The drawing under review shows one solid part. Ordinate dimensions are in mm from its lowest x, y, z. Round coordinates to 2 decimals unless told otherwise and drop trailing zeros. Write each loop counter-clockwise with the first axis right and the second up, starting at its lowest first coordinate (ties: lowest second). Pieces come first, ordered by that corner, then holes. Notation, with made-up numbers: (86.5, 61.5) -> (138.5, 61.5) arc R20 cw to (138.5, 86.5) -> close; hole circle Ø8 at (45.25, 70.5). An arc over 180 degrees is marked (long way). Write item = value, one per line. Start each with the question number.
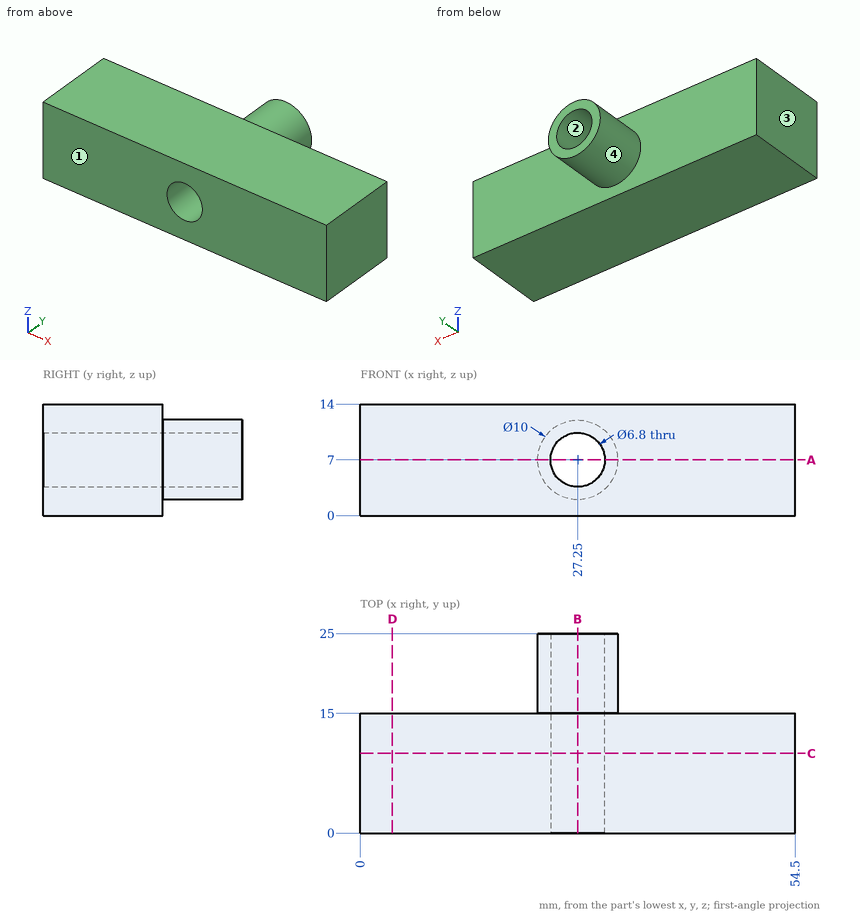
1. Draft analysis for pull direction X (two halves, no side actions). For the marked faces 1, 2, 3 and 4, state which applies: +X half, -X half, draft (parallel to the pull), parting line (faces both ways), or undercut.
2. Consider section B-B, the plane x = 27.25. Give the boundary of the cut face in (y, z).
3. Wall thickness on L1, parallel to Z at x = 27.25, y = 19; L2, parallel to X at y = 23.5, z = 7.25; L3, parallel to Z at x = 27.25, y = 5.5: over which ranges is each line inside the solid? List them lowest first. Write a range as from..to.
4. Consider section D-D, the plane x = 4. Give the boundary of the cut face in (y, z), then the cut area to 3 significant figures.
5. Clearance check with flat-ended pins moving along their axes: pin 1 Ø1 at (y, z) = (16.5, 6) entering from +X; pin 2 Ø3 at (x, z) = (16.5, 2.5) entering from +Y; pin 3 Ø5.5 at (x, z) = (27.25, 7) entering from -Y. State where each tip first meets the part, or that it passes through.
6. Consider section A-A, the plane z = 7. Give the boundary of the cut face in (x, y).
7. Consider section C-C, the plane y = 10. Give the boundary of the cut face in (x, z).
Outcome:
q1.face_1 = draft
q1.face_2 = undercut
q1.face_3 = -X half
q1.face_4 = parting line
q2.outline = (0, 0) -> (15, 0) -> (15, 2) -> (25, 2) -> (25, 3.6) -> (0, 3.6) -> close; (0, 10.4) -> (25, 10.4) -> (25, 12) -> (15, 12) -> (15, 14) -> (0, 14) -> close
q3.L1 = 2..3.6, 10.4..12
q3.L2 = 22.26..23.86, 30.64..32.24
q3.L3 = 0..3.6, 10.4..14
q4.outline = (0, 0) -> (15, 0) -> (15, 14) -> (0, 14) -> close
q4.area = 210 mm2
q5.pin_1 = 32.22
q5.pin_2 = 15
q5.pin_3 = through
q6.outline = (0, 0) -> (23.85, 0) -> (23.85, 25) -> (22.25, 25) -> (22.25, 15) -> (0, 15) -> close; (30.65, 0) -> (54.5, 0) -> (54.5, 15) -> (32.25, 15) -> (32.25, 25) -> (30.65, 25) -> close
q7.outline = (0, 0) -> (54.5, 0) -> (54.5, 14) -> (0, 14) -> close; hole circle Ø6.8 at (27.25, 7)
